Source: three-view drawing plus pictorial views. Frame: mm from the lowest corner of the part. A direction names the side the tool comes from. Round coordinates to 2 decimals unless told otherwise and drop trailing zeros. Order: outer loops, then holes, each group sorted by start corner. A loop starts at its lowest first (then second) coordinate and runs counter-clockwise, first axis right, second up. Notation, with made-up numbers: (86, -12) -> (107, -12) arc R19 cw to (107, -6) -> close; hole circle Ø7 at (-9.75, 1.25). An arc over 180 degrees is marked (long way). Use a Markdown table: item, result.
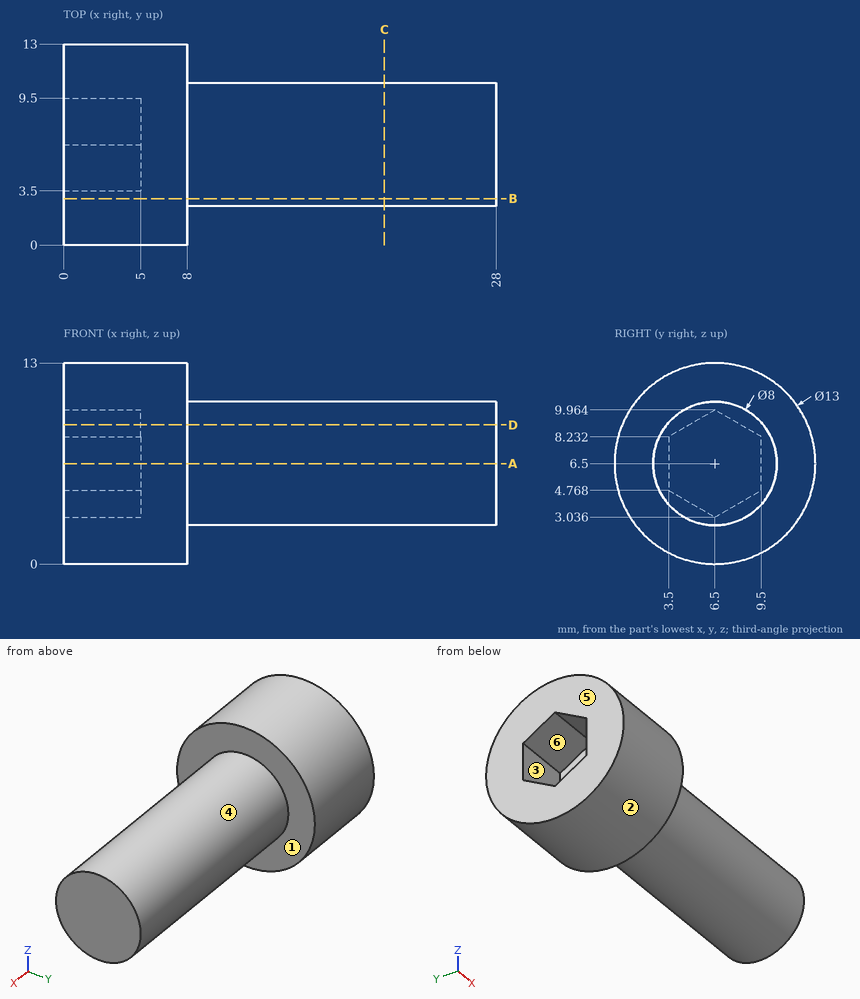
1) Pull-direction query (Z, two-part tool) for the marked faces 4, 5 and 6; classes: +Z half, -Z half, draft (parallel to the pull), parting line (faces both ways), or undercut.
Results found:
| item | result |
|---|---|
| face 4 | parting line |
| face 5 | draft |
| face 6 | undercut |
2) Cut plane B-B on y = 3. Return loops of the section in (x, z), and give its area (3 significant figures).
Results found:
| item | result |
|---|---|
| outline | (0, 1.02) -> (8, 1.02) -> (8, 4.56) -> (28, 4.56) -> (28, 8.44) -> (8, 8.44) -> (8, 11.98) -> (0, 11.98) -> close |
| area | 165 mm² |
3) Cut plane D-D on z = 9. Return loops of the section in (x, y).
Results found:
| item | result |
|---|---|
| outline | (0, 0.5) -> (8, 0.5) -> (8, 3.38) -> (28, 3.38) -> (28, 9.62) -> (8, 9.62) -> (8, 12.5) -> (0, 12.5) -> (0, 8.17) -> (5, 8.17) -> (5, 4.83) -> (0, 4.83) -> close |
4) Line query: L1, parallel to Y at x = 17.75, z = 6.5; L2, parallel to X at y = 11, z = 7; L3, parallel to Y at x = 3.5, z = 8.75. Output: solid intervals per line, ascending. Write a range as [from, to].
Results found:
| item | result |
|---|---|
| L1 | y = [2.5, 10.5] |
| L2 | x = [0, 8] |
| L3 | y = [0.4, 4.4], [8.6, 12.6] |
5) Pin query (flat end, axial travel): pin 1 Ø3 at (y, z) = (7.5, 6.5) entering from -X; pin 2 Ø1.5 at (x, y) = (9.5, 3) entering from -Z (1 decimal); pin 3 Ø4 at (x, z) = (20.5, 7.5) entering from -Y. Return the tip coordinate at first contact, or that it passes through.
Results found:
| item | result |
|---|---|
| pin 1 | stops at x = 5 |
| pin 2 | stops at z = 3.6 |
| pin 3 | stops at y = 2.5 |
6) Cut plane C-C on x = 20.75. Return loops of the section in (y, z), and give its area (3 significant figures).
Results found:
| item | result |
|---|---|
| outline | circle Ø8 at (6.5, 6.5) |
| area | 50.3 mm² |
7) Cut plane A-A on z = 6.5. Return loops of the section in (x, y), and give its area (3 significant figures).
Results found:
| item | result |
|---|---|
| outline | (0, 0) -> (8, 0) -> (8, 2.5) -> (28, 2.5) -> (28, 10.5) -> (8, 10.5) -> (8, 13) -> (0, 13) -> (0, 9.5) -> (5, 9.5) -> (5, 3.5) -> (0, 3.5) -> close |
| area | 234 mm² |
8) Set-up query: the marked faces 1, 2 and 3. Return all of +Z, -Z, +X, -X, +Y, -Y with unobstructed straight access to the full face (end or side cutting, diameter ignored); none if empty.
Results found:
| item | result |
|---|---|
| face 1 | +X |
| face 2 | +X, -X |
| face 3 | -X |
